from build123d import *

# Parameters (mm, degrees)
SKETCH1_R           = 3
BOSS_EXTRUDE2_DEPTH = 5


with BuildPart() as part:
    # Sketch1 → Boss-Extrude2 (new body)
    with BuildSketch(Plane.XY):
        with BuildLine():
            ThreePointArc((-19.550519413, 15.581309017), (-18.238129642, 12.880402273), (-16.110253623, 10.761580005))
            ThreePointArc((-16.110253623, 10.761580005), (-16.778376173, 9.687), (-17.374928481, 8.571098896))
            ThreePointArc((-17.374928481, 8.571098896), (-20.2738204, 9.354482451), (-23.269069139, 9.14059196))
            ThreePointArc((-23.269069139, 9.14059196), (-23.49231552, 8.550503583), (-23.700600368, 7.954969654))
            ThreePointArc((-23.700600368, 7.954969654), (-21.543592873, 5.865811255), (-18.819363584, 4.602546066))
            ThreePointArc((-18.819363584, 4.602546066), (-19.079665407, 3.364259794), (-19.258580553, 2.111622855))
            ThreePointArc((-19.258580553, 2.111622855), (-22.250580854, 1.856283171), (-24.992039135, 0.630856452))
            ThreePointArc((-24.992039135, 0.630856452), (-25, 0), (-24.992039135, -0.630856452))
            ThreePointArc((-24.992039135, -0.630856452), (-22.250580854, -1.856283171), (-19.258580553, -2.111622855))
            ThreePointArc((-19.258580553, -2.111622855), (-19.079665407, -3.364259794), (-18.819363584, -4.602546066))
            ThreePointArc((-18.819363584, -4.602546066), (-21.543592873, -5.865811255), (-23.700600368, -7.954969654))
            ThreePointArc((-23.700600368, -7.954969654), (-23.49231552, -8.550503583), (-23.269069139, -9.14059196))
            ThreePointArc((-23.269069139, -9.14059196), (-20.2738204, -9.354482451), (-17.374928481, -8.571098896))
            ThreePointArc((-17.374928481, -8.571098896), (-16.778376173, -9.687), (-16.110253623, -10.761580005))
            ThreePointArc((-16.110253623, -10.761580005), (-18.238129642, -12.880402273), (-19.550519413, -15.581309017))
            ThreePointArc((-19.550519413, -15.581309017), (-19.151111078, -16.069690242), (-18.739505991, -16.547837177))
            ThreePointArc((-18.739505991, -16.547837177), (-15.851737997, -15.724393089), (-13.395603607, -13.996773914))
            ThreePointArc((-13.395603607, -13.996773914), (-12.45336715, -14.841345041), (-11.458009312, -15.622608572))
            ThreePointArc((-11.458009312, -15.622608572), (-12.73287881, -18.341426683), (-13.042357282, -21.328312557))
            ThreePointArc((-13.042357282, -21.328312557), (-12.5, -21.650635095), (-11.949681854, -21.95916901))
            ThreePointArc((-11.949681854, -21.95916901), (-9.517702044, -20.197709854), (-7.800571241, -17.734231427))
            ThreePointArc((-7.800571241, -17.734231427), (-6.626298257, -18.205604835), (-5.423759977, -18.59931998))
            ThreePointArc((-5.423759977, -18.59931998), (-5.691854876, -21.590204344), (-4.961094377, -24.502806831))
            ThreePointArc((-4.961094377, -24.502806831), (-4.341204442, -24.620193825), (-3.718549727, -24.721900977))
            ThreePointArc((-3.718549727, -24.721900977), (-2.035690758, -22.234884724), (-1.264674858, -19.332678901))
            ThreePointArc((-1.264674858, -19.332678901), (0, -19.374), (1.264674858, -19.332678901))
            ThreePointArc((1.264674858, -19.332678901), (2.035690758, -22.234884724), (3.718549727, -24.721900977))
            ThreePointArc((3.718549727, -24.721900977), (4.341204442, -24.620193825), (4.961094377, -24.502806831))
            ThreePointArc((4.961094377, -24.502806831), (5.691854876, -21.590204344), (5.423759977, -18.59931998))
            ThreePointArc((5.423759977, -18.59931998), (6.626298257, -18.205604835), (7.800571241, -17.734231427))
            ThreePointArc((7.800571241, -17.734231427), (9.517702044, -20.197709854), (11.949681854, -21.95916901))
            ThreePointArc((11.949681854, -21.95916901), (12.5, -21.650635095), (13.042357282, -21.328312557))
            ThreePointArc((13.042357282, -21.328312557), (12.73287881, -18.341426683), (11.458009312, -15.622608572))
            ThreePointArc((11.458009312, -15.622608572), (12.45336715, -14.841345041), (13.395603607, -13.996773914))
            ThreePointArc((13.395603607, -13.996773914), (15.851737997, -15.724393089), (18.739505991, -16.547837177))
            ThreePointArc((18.739505991, -16.547837177), (19.151111078, -16.069690242), (19.550519413, -15.581309017))
            ThreePointArc((19.550519413, -15.581309017), (18.238129642, -12.880402273), (16.110253623, -10.761580005))
            ThreePointArc((16.110253623, -10.761580005), (16.778376173, -9.687), (17.374928481, -8.571098896))
            ThreePointArc((17.374928481, -8.571098896), (20.2738204, -9.354482451), (23.269069139, -9.14059196))
            ThreePointArc((23.269069139, -9.14059196), (23.49231552, -8.550503583), (23.700600368, -7.954969654))
            ThreePointArc((23.700600368, -7.954969654), (21.543592873, -5.865811255), (18.819363584, -4.602546066))
            ThreePointArc((18.819363584, -4.602546066), (19.079665407, -3.364259794), (19.258580553, -2.111622855))
            ThreePointArc((19.258580553, -2.111622855), (22.250580854, -1.856283171), (24.992039135, -0.630856452))
            ThreePointArc((24.992039135, -0.630856452), (25, 0), (24.992039135, 0.630856452))
            ThreePointArc((24.992039135, 0.630856452), (22.250580854, 1.856283171), (19.258580553, 2.111622855))
            ThreePointArc((19.258580553, 2.111622855), (19.079665407, 3.364259794), (18.819363584, 4.602546066))
            ThreePointArc((18.819363584, 4.602546066), (21.543592873, 5.865811255), (23.700600368, 7.954969654))
            ThreePointArc((23.700600368, 7.954969654), (23.49231552, 8.550503583), (23.269069139, 9.14059196))
            ThreePointArc((23.269069139, 9.14059196), (20.2738204, 9.354482451), (17.374928481, 8.571098896))
            ThreePointArc((17.374928481, 8.571098896), (16.778376173, 9.687), (16.110253623, 10.761580005))
            ThreePointArc((16.110253623, 10.761580005), (18.238129642, 12.880402273), (19.550519413, 15.581309017))
            ThreePointArc((19.550519413, 15.581309017), (19.151111078, 16.069690242), (18.739505991, 16.547837177))
            ThreePointArc((18.739505991, 16.547837177), (15.851737997, 15.724393089), (13.395603607, 13.996773914))
            ThreePointArc((13.395603607, 13.996773914), (12.45336715, 14.841345041), (11.458009312, 15.622608572))
            ThreePointArc((11.458009312, 15.622608572), (12.73287881, 18.341426683), (13.042357282, 21.328312557))
            ThreePointArc((13.042357282, 21.328312557), (12.5, 21.650635095), (11.949681854, 21.95916901))
            ThreePointArc((11.949681854, 21.95916901), (9.517702044, 20.197709854), (7.800571241, 17.734231427))
            ThreePointArc((7.800571241, 17.734231427), (6.626298257, 18.205604835), (5.423759977, 18.59931998))
            ThreePointArc((5.423759977, 18.59931998), (5.691854876, 21.590204344), (4.961094377, 24.502806831))
            ThreePointArc((4.961094377, 24.502806831), (4.341204442, 24.620193825), (3.718549727, 24.721900977))
            ThreePointArc((3.718549727, 24.721900977), (2.035690758, 22.234884724), (1.264674858, 19.332678901))
            ThreePointArc((1.264674858, 19.332678901), (0, 19.374), (-1.264674858, 19.332678901))
            ThreePointArc((-1.264674858, 19.332678901), (-2.035690758, 22.234884724), (-3.718549727, 24.721900977))
            ThreePointArc((-3.718549727, 24.721900977), (-4.341204442, 24.620193825), (-4.961094377, 24.502806831))
            ThreePointArc((-4.961094377, 24.502806831), (-5.691854876, 21.590204344), (-5.423759977, 18.59931998))
            ThreePointArc((-5.423759977, 18.59931998), (-6.626298257, 18.205604835), (-7.800571241, 17.734231427))
            ThreePointArc((-7.800571241, 17.734231427), (-9.517702044, 20.197709854), (-11.949681854, 21.95916901))
            ThreePointArc((-11.949681854, 21.95916901), (-12.5, 21.650635095), (-13.042357282, 21.328312557))
            ThreePointArc((-13.042357282, 21.328312557), (-12.73287881, 18.341426683), (-11.458009312, 15.622608572))
            ThreePointArc((-11.458009312, 15.622608572), (-12.45336715, 14.841345041), (-13.395603607, 13.996773914))
            ThreePointArc((-13.395603607, 13.996773914), (-15.851737997, 15.724393089), (-18.739505991, 16.547837177))
            ThreePointArc((-18.739505991, 16.547837177), (-19.151111078, 16.069690242), (-19.550519413, 15.581309017))
        make_face()
        Circle(SKETCH1_R, mode=Mode.SUBTRACT)
    extrude(amount=BOSS_EXTRUDE2_DEPTH)


solid = part.part
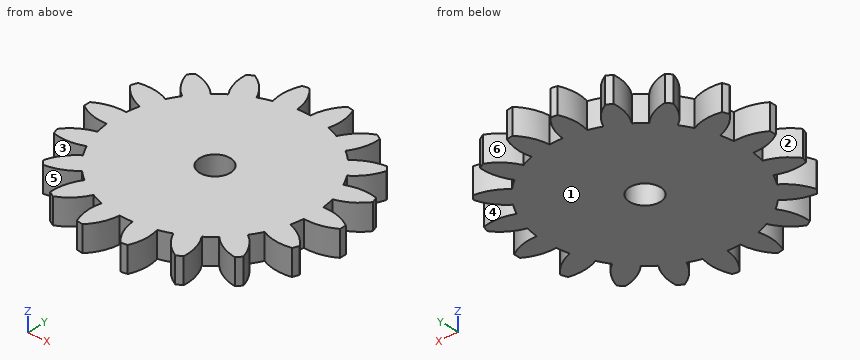
The model under review builds one solid part; all positions refer to its coordinate system, in mm. Face numbers are marked on the shaded views. A direction names the side the tool comes from. Round coordinates to 2 decimals unless told otherwise and drop trailing zeros. Loops run counter-clockwise (first coordinate to the right, second up) from the corner with the lowest first, then second, coordinate; pieces in that order, holes last. Notation, with made-up numbers: M -2.75,57 L 17.25,57 A14 cw 17.25,78 Z; hole C -38.75,-36.5 d5. An arc over 180 degrees is marked long. Answer as CSV lines item,"result".
1. Draft analysis for pull direction X (two halves, no side actions). For the marked faces 1, 2 and 3, state which applies: pulls with the +X half, pulls with the -X half, needs draft (parallel to the pull), parting line crosses it, or undercut.
Outcome:
face 1,"needs draft"
face 2,"pulls with the -X half"
face 3,"undercut"
2. We need section C-C (y = -15). Give the boundary of the cut face in (x, z).
Outcome:
outline,"M -19.36,0 L -14.6,0 L -14.6,5 L -19.36,5 Z; M -12.26,0 L 12.26,0 L 12.26,5 L -12.26,5 Z; M 14.6,0 L 19.36,0 L 19.36,5 L 14.6,5 Z"
3. We need section A-A (x = 0). Give the boundary of the cut face in (y, z).
Outcome:
outline,"M -19.37,0 L -3,0 L -3,5 L -19.37,5 Z; M 3,0 L 19.37,0 L 19.37,5 L 3,5 Z"
4. Insertion check: pin 1 Ø3 at (y, z) = (14.5, 4) entering from +X; pin 2 Ø2 at (x, z) = (19, 3) entering from -Y; pin 3 Ø3.5 at (x, y) = (0, 0) entering from -Z. Each pin has a flat end and moves straight along its axis. Give the tip position at first contact, or say it passes through.
Outcome:
pin 1,"stops at x = 19.55"
pin 2,"stops at y = -16.55"
pin 3,"passes through"
5. We need section B-B (y = 0). Give the boundary of the cut face in (x, z).
Outcome:
outline,"M -25,0 L -3,0 L -3,5 L -25,5 Z; M 3,0 L 25,0 L 25,5 L 3,5 Z"
6. To check wall thickness, follow L1, parallel to Y at x = 0, z = 1.15; L2, parallel to X at y = 19, z = 3.1; L3, parallel to Y at x = 21.5, z = 1.5. State the ranges of each line that lie inside material, in increasing order. Write a range as [from, to].
Outcome:
L1,"y = [-19.37, -3], [3, 19.37]"
L2,"x = [-12.89, -8.53], [-5.52, 5.52], [8.53, 12.89]"
L3,"y = [-9.39, -5.84], [-2.02, 2.02], [5.84, 9.39]"
7. We need section D-D (x = -14). Give the boundary of the cut face in (y, z), plus the area to 3 significant figures.
Outcome:
outline,"M -14.54,0 L 14.54,0 L 14.54,5 L -14.54,5 Z"
area,"145 mm2"
8. For the marked faces 4, 5 and 6, list the 3-axis set-ups (+Z, -Z, +X, -X, +Y, -Y) from which the entire face can be reached by the end or side of a thin tool; tool diameter is ignored.
Outcome:
face 4,"+Z, -Z"
face 5,"+Z, -Z, -Y"
face 6,"+Z, -Z, +Y"
